Geometry check sheet. Reference: the model listing, model coordinates, mm. A direction names the side the tool comes from. Give positions to 0.01 mm unless a question says otherwise; leave off trailing zeros. Order: outer loops, then holes, each group sorted by start corner. A loop starts at its lowest first (then second) coordinate and runs counter-clockwise, first axis right, second up.
```python
from build123d import *

# Parameters (mm, degrees)
BOSS_EXTRUDE1_DEPTH  = 160
M4_CLEARANCE_HOLE1_D = 4.5
CUT_EXTRUDE2_REACH   = 163.357
SKETCH5_R            = 3.1


with BuildPart() as part:
    # Sketch1 → Boss-Extrude1 (new body)
    with BuildSketch(Plane.XY):
        Polygon((4, -4), (16, -4), (16, -10), (20, -10), (20, 0), (16, 0), (4, 0), align=None)
    extrude(amount=BOSS_EXTRUDE1_DEPTH)

    # M4 Clearance Hole1 (through all)
    with Locations(Plane(origin=(0, -4, 0), x_dir=(-1, 0, 0), z_dir=(0, -1, 0))):
        with Locations((-10.128911503, -6.267286375), (-10.128911503, -23.38156703), (-10.128911503, -42.093180546), (-10.128911503, -63.314888558), (-9.444340277, -107.583827852), (-9.444340277, -150.244789298)):
            Hole(M4_CLEARANCE_HOLE1_D / 2)

    # Sketch5 → Cut-Extrude2 (cut, up to next)
    with BuildSketch(Plane.XZ.offset(4), mode=Mode.PRIVATE) as cut_extrude2_sk1:
        with Locations(Location((9, 138.897931951, 0), (0, 0, 270))):
            Circle(SKETCH5_R)
    cut_extrude2_tool1 = extrude(cut_extrude2_sk1.sketch, amount=-CUT_EXTRUDE2_REACH, mode=Mode.PRIVATE) & part.part
    add(cut_extrude2_tool1.solids().sort_by_distance((9, -4, 138.897932))[0], mode=Mode.SUBTRACT)


solid = part.part
```
Q1. Cross-section at B-B, the plane y = -8.25. Record the boundary of the cut face in (x, z).
Q2. Thickness scan on L1, parallel to Y at x = 13.25, z = 77.5; L2, parallel to Z at x = 7.5, y = -0.75 (3 decimals); L3, parallel to Z at x = 7, y = -3. Record the ranges inside material, lowest first.
Q3. Release check for a two-part mould opening along Z. For faces 1 (the face through (14, -3, 160)), 2 (the face through (9.641, -1.972, 25.578)), 3 (the face through (10, -4, 79)) record: pulls with the +Z half, pulls with the -Z half, needs draft (parallel to the pull), parting line crosses it, or undercut.
Q4. Cross-section at A-A, the plane z = 77. Record the boundary of the cut face in (x, y), and give its area (3 significant figures).
Q5. Gauge pin test, flat ends, axial feed: P1, Ø5, axis at x = 6.5, z = 65.5, coming from the +Y side; P2, Ø1.5, axis at x = 12.5, z = 108.5, coming from the -Y side. Record the tip position at first contact, or that the pin passes through.
Q6. Access from +Z, -Z, +X, -X, +Y, -Y to the whole of each face (thin tool, end or side, straight path). Record for faces 4 (the face through (9.84, -1.97, 39.86)), 5 (the face through (16, -7, 79)).
Answers follow:
1. outline: (16, 0) - (20, 0) - (20, 160) - (16, 160) - close
2. L1: y = -4 to 0
2. L2: z = 0 to 106.452, 108.716 to 136.185, 141.611 to 149.113, 151.377 to 160
2. L3: z = 0 to 136.53, 141.27 to 160
3. face 1: pulls with the +Z half
3. face 2: undercut
3. face 3: needs draft
4. outline: (4, -4) - (16, -4) - (16, -10) - (20, -10) - (20, 0) - (4, 0) - close
4. area: 88.0 mm2
5. P1: stops at y = 0
5. P2: stops at y = -4
6. face 4: +Y, -Y
6. face 5: +Z, -Z, -X, -Y
